from build123d import *

# Parameters (mm, degrees)
CUT_EXTRUDE_1_DEPTH      = 18.972200756
CUT_EXTRUDE_1_DEPTH_BACK = 18.972200756
SKETCH_2_W               = 3.275
SKETCH_2_H               = 4
SKETCH_3_R               = 4
CUT_EXTRUDE_2_DEPTH      = 4
CHAMFER_1_SIZE           = 1
CHAMFER_2_SIZE           = 0.2


with BuildPart() as part:
    # Эскиз1 → Повернуть1 (revolve)
    with BuildSketch(Plane(origin=(0, 0, 0), x_dir=(0, 0, -1), z_dir=(1, 0, 0)), mode=Mode.PRIVATE) as revolve_1_sk:
        Polygon((3.5, 15), (3.5, 0), (5.175, 0), (5.175, 11), (7, 11), (7, 15), align=None)
    revolve(revolve_1_sk.sketch.rotate(Axis((0, 26.762195122, 0), (0, -1, 0)), 180), axis=Axis((0, 26.762195122, 0), (0, -1, 0)))

    # Эскиз2 → Вырез-Вытянуть1 (cut, two sides: drawn at the far end of the back side and taken through both)
    with BuildSketch(Plane.XY.offset(-CUT_EXTRUDE_1_DEPTH_BACK)):
        with Locations((3.5375, 2)):
            Rectangle(SKETCH_2_W, SKETCH_2_H)
        with Locations((-3.5375, 2)):
            Rectangle(SKETCH_2_W, SKETCH_2_H)
    extrude(amount=CUT_EXTRUDE_1_DEPTH + CUT_EXTRUDE_1_DEPTH_BACK, mode=Mode.SUBTRACT)

    # Эскиз3 → Вырез-Вытянуть2 (cut)
    with BuildSketch(Plane.XZ.offset(-4)):
        Circle(SKETCH_3_R)
    extrude(amount=CUT_EXTRUDE_2_DEPTH, mode=Mode.SUBTRACT)

    # Фаска1
    # the kernel refuses this chamfer: 1 mm, written as the material it takes off along each edge
    with BuildSketch(Plane(origin=(0, 4, 0), x_dir=(0, 0, 1), z_dir=(1, 0, 0))) as chamfer_1_piece_1_section:
        Polygon((3.5, -CHAMFER_1_SIZE), (3.5 + CHAMFER_1_SIZE, 0), (3.5, 0), align=None)
    chamfer_1_piece_1 = revolve(axis=Axis((0, 4, 0), (0, -1, 0)), mode=Mode.PRIVATE)
    chamfer_1_piece_1 = chamfer_1_piece_1 & Plane(origin=(0, 4.334033243, 0), x_dir=(1, 0, 0), z_dir=(0, 1, 0)) * Cylinder(4, 19, mode=Mode.PRIVATE)
    add(chamfer_1_piece_1, mode=Mode.SUBTRACT)
    with BuildSketch(Plane(origin=(0, 4, 0), x_dir=(0, 0, 1), z_dir=(1, 0, 0))) as chamfer_1_piece_2_section:
        Polygon((3.5, -CHAMFER_1_SIZE), (3.5 + CHAMFER_1_SIZE, 0), (3.5, 0), align=None)
    chamfer_1_piece_2 = revolve(axis=Axis((0, 4, 0), (0, -1, 0)), mode=Mode.PRIVATE)
    chamfer_1_piece_2 = split(chamfer_1_piece_2, bisect_by=Plane(origin=(-1.9, 4.24260685, 0), z_dir=(-1, 0, 0)), keep=Keep.TOP, mode=Mode.PRIVATE)
    add(chamfer_1_piece_2, mode=Mode.SUBTRACT)
    with BuildSketch(Plane(origin=(0, 4, 0), x_dir=(0, 0, 1), z_dir=(1, 0, 0))) as chamfer_1_piece_3_section:
        Polygon((3.5, -CHAMFER_1_SIZE), (3.5 + CHAMFER_1_SIZE, 0), (3.5, 0), align=None)
    chamfer_1_piece_3 = revolve(axis=Axis((0, 4, 0), (0, -1, 0)), mode=Mode.PRIVATE)
    chamfer_1_piece_3 = split(chamfer_1_piece_3, bisect_by=Plane(origin=(1.9, 4.24260685, 0), z_dir=(1, 0, 0)), keep=Keep.TOP, mode=Mode.PRIVATE)
    add(chamfer_1_piece_3, mode=Mode.SUBTRACT)
    with BuildSketch(Plane(origin=(0, 15, 0), x_dir=(0, 0, 1), z_dir=(1, 0, 0))) as chamfer_1_piece_4:
        Polygon((3.5, CHAMFER_1_SIZE), (3.5 + CHAMFER_1_SIZE, 0), (3.5, 0), align=None)
    revolve(axis=Axis((0, 15, 0), (0, -1, 0)), mode=Mode.SUBTRACT)

    # Фаска2
    chamfer_2_edges = [part.edges().sort_by_distance(p)[0] for p in [
        (0, 0, -5.175),
        (5.175, 4, 0),
        (0.967033992, 0, 5.083844043),
        (-5.175, 4, 0),
        (0, 15, -7),
        (0, 11, -7),
        (0, 11, -5.175),
        (0, 0, -4),
        (0, 0, 4),
    ]]
    chamfer(chamfer_2_edges, length=CHAMFER_2_SIZE)


solid = part.part
Could you check a few things on this model? Use its own coordinates, in mm. A direction names the side the tool comes from. Round coordinates to 2 decimals unless told otherwise and drop trailing zeros. Write each loop counter-clockwise with the first axis right and the second up, starting at its lowest first coordinate (ties: lowest second). Pieces come first, ordered by that corner, then holes. Notation, with made-up numbers: (19, 67.5) - (73, 67.5) arc R23 ccw to (73, 96.5) - close; hole circle Ø3 at (-6, 43.5). An arc over 180 degrees is marked (long way). Put each result on its own line as item: value. Start each with the question number.
(1) Will these pins go through, and if not, where does the flat tip stop? pin 1 (4 mm diameter, centred on x = 4, z = -1.5, fed in from +Y); pin 2 (1.4 mm diameter, centred on y = 2.5, z = 4, fed in from +X); pin 3 (5 mm diameter, centred on y = 13, z = 3, fed in from +X); pin 4 (0.9 mm diameter, centred on x = 3, z = 0, fed in from -Y).
(2) For faces 4 (the flat face through (0, 0, -4.5)), 5 (the cylindrical face through (0, 2, 4)), 6 (the flat face through (-4.7, 4, 0.4)), which set-ups out of +Z, -Z, +X, -X, +Y, -Y let a thin tool reach every point of the face, with its end or its side?
(3) Thinking about a two-plate mould opening in Z: for faces 1 (the cylindrical face through (0, 2, -4)), 2 (the cylindrical face through (2.681, 13.025, 6.466)), 3 (the flat face through (4.7, 4, 0)), which applies, released by +Z, released by -Z, zero draft, split by the parting line, or undercut?
(4) I need wall thicknesses on probe 1 along X at (y, z) = (9.5, 0) (3 decimals); probe 2 along X at (y, z) = (11.75, 0); probe 3 along Y at (x, z) = (3.5, -2.5). Which ranges of each line are inside material? Lowest first, please.
(5) I want a section at C-C, the plane x = 0. Please give me the cut outline in (y, z) (3 decimals).
(6) I want a section at D-D, the plane y = 6. Please give me the cut outline in (x, z) (3 decimals).
(7) I want a section at A-A, the plane z = 0. Please give me the cut outline in (x, y) (3 decimals).
(8) I want a section at B-B, the plane y = 3.5. Please give me the cut outline in (x, z) (3 decimals).
Here are the results:
1. pin 1: stops at y = 15
1. pin 2: stops at x = 1.9
1. pin 3: stops at x = 6.98
1. pin 4: passes through
2. face 4: +Z, -Z, +X, -X, -Y
2. face 5: -Y
2. face 6: +Z, -Z, -X, -Y
3. face 1: undercut
3. face 2: split by the parting line
3. face 3: zero draft
4. probe 1: x = -5.175 to -3.5, 3.5 to 5.175
4. probe 2: x = -7 to -3.5, 3.5 to 7
4. probe 3: y = 4.2 to 14.8
5. outline: (0, -4.975) - (0.2, -5.175) - (10.8, -5.175) - (11, -5.375) - (11, -6.8) - (11.2, -7) - (14.8, -7) - (15, -6.8) - (15, -4.5) - (14, -3.5) - (5, -3.5) - (4.5, -4) - (0.2, -4) - (0, -4.2) - close; (0, 4.2) - (0.2, 4) - (4.5, 4) - (5, 3.5) - (14, 3.5) - (15, 4.5) - (15, 6.8) - (14.8, 7) - (11.2, 7) - (11, 6.8) - (11, 5.375) - (10.8, 5.175) - (0.2, 5.175) - (0, 4.975) - close
6. outline: circle Ø10.35 at (0, 0); hole circle Ø7 at (0, 0)
7. outline: (-7, 11.2) - (-6.8, 11) - (-5.375, 11) - (-5.175, 10.8) - (-5.175, 4.2) - (-4.975, 4) - (-4.5, 4) - (-3.5, 5) - (-3.5, 14) - (-4.5, 15) - (-6.8, 15) - (-7, 14.8) - close; (3.5, 5) - (4.5, 4) - (4.975, 4) - (5.175, 4.2) - (5.175, 10.8) - (5.375, 11) - (6.8, 11) - (7, 11.2) - (7, 14.8) - (6.8, 15) - (4.5, 15) - (3.5, 14) - close
8. outline: (-1.9, -4.814) arc R5.175 ccw to (1.9, -4.814) - (1.9, -3.52) arc R4 cw to (-1.9, -3.52) - close; (-1.9, 3.52) arc R4 cw to (1.9, 3.52) - (1.9, 4.814) arc R5.175 ccw to (-1.9, 4.814) - close
